Work out the finished part from the listing and answer in its coordinate system (mm). Coordinates: 2 decimals unless noted, no trailing zeros. Order: outer loops, then holes, each group sorted by start corner. A loop starts at its lowest first (then second) coordinate and runs counter-clockwise, first axis right, second up.
1. Determine the mould class of faces 1 (the flat face through (0, 1, -12.25)), 2 (the cylindrical face through (-0.046, 1.014, 6.457)), 3 (the flat face through (-12.25, 1, 0)) for opening direction Z: +Z half, -Z half, draft (parallel to the pull), parting line (faces both ways), or undercut.
2. The part is cut by section C-C, the plane y = 1. Give the vertices of the cut face in (x, z).
3. Find the intervals of material crossed by probe 1 along Z at (x, y) = (0, 0.4); probe 2 along X at (y, z) = (0.9, 0); probe 3 along Z at (x, y) = (-0.5, 1.8), in increasing order.
4. The part is cut by section A-A, the plane z = 0. Give the vertices of the cut face in (x, y).
5. The part is cut by section B-B, the plane x = 0. Give the vertices of the cut face in (y, z), then the cut area to 3 significant figures.
6. A flat-ended cylindrical pin translates along its axis: pin 1 Ø13.5 at (x, z) = (0, 0) entering from +Y. Find the tip coordinate at first contact, or state that the pin passes through.
Autodesk Inventor part; units mm, degrees
ref_plane "YZ Plane" through (0, 0, 0) normal (1, 0, 0) x (0, 1, 0)
ref_plane "XZ Plane" through (0, 0, 0) normal (0, 1, 0) x (-1, 0, 0)
ref_plane "XY Plane" through (0, 0, 0) normal (0, 0, 1) x (1, 0, 0)
sketch "Sketch1" plane through (0, 0, 0) normal (0, 1, 0) x (-1, 0, 0)
  circle A0 centre (0, 0) radius 4.25
  line L0 (-12.25, -12.25) -> (12.25, -12.25)
  line L1 (12.25, -12.25) -> (12.25, 12.25)
  line L2 (12.25, 12.25) -> (-12.25, 12.25)
  line L3 (-12.25, 12.25) -> (-12.25, -12.25)
  line L4 (-12.25, -12.25) -> (12.25, 12.25) construction
  line L5 (12.25, -12.25) -> (-12.25, 12.25) construction
  dimension "d0" = 24.5
  dimension "d1" = 8.5
extrude "Extrusion1" add sketch "Sketch1" along normal blind 2
sketch "Sketch2" plane through (0, 2, 0) normal (0, 1, 0) x (1, 0, 0)
  circle A0 centre (0, -4.9582) radius 1.5
  point P0 (0, 0)
  dimension "d4" = 3
extrude "Extrusion2" cut sketch "Sketch2" against normal blind 3
equation "\"d5\" = d4"
properties part number "pb_hole" material "Lead"
Geometry says:
1. face 1: -Z half
1. face 2: undercut
1. face 3: draft
2. outline: (-12.25, -12.25) - (12.25, -12.25) - (12.25, 12.25) - (-12.25, 12.25) - close; hole (-1.21, 4.07) arc R4.25 ccw (long way) to (1.21, 4.07) arc R1.5 ccw (long way) to start
3. probe 1: z = -12.25 to -4.25, 6.46 to 12.25
3. probe 2: x = -12.25 to -4.25, 4.25 to 12.25
3. probe 3: z = -12.25 to -4.22, 6.37 to 12.25
4. outline: (-12.25, 0) - (-4.25, 0) - (-4.25, 2) - (-12.25, 2) - close; (4.25, 0) - (12.25, 0) - (12.25, 2) - (4.25, 2) - close
5. outline: (0, -12.25) - (2, -12.25) - (2, -4.25) - (0, -4.25) - close; (0, 6.46) - (2, 6.46) - (2, 12.25) - (0, 12.25) - close
5. area: 27.6 mm2
6. pin 1: stops at y = 2
